from build123d import *

# Parameters (mm, degrees)
BOSS_EXTRUDE1_DEPTH = 8.89
CHAMFER1_SIZE       = 7.46
CHAMFER1_SIZE2      = 42.307762374


with BuildPart() as part:
    # Sketch2 → Boss-Extrude1 (new body)
    with BuildSketch(Plane(origin=(0, 0, 0), x_dir=(1, 0, 0), z_dir=(0, 1, 0))):
        Polygon((133.286430852, -770.74001749), (147.934191067, -816.056525657), (356.664774137, -778.521640105), (352.263248298, -717.230631168), align=None)
    extrude(amount=-BOSS_EXTRUDE1_DEPTH)

    # Chamfer1
    chamfer1_edges = [part.edges().sort_by_distance(p)[0] for p in [
        (252.299482602, 0, 797.289082881),
    ]]
    chamfer1_side = [part.faces().sort_by_distance(p)[0] for p in [
        (252.299482602, -4.445, 797.289082881),
    ]]
    chamfer(chamfer1_edges, length=CHAMFER1_SIZE, length2=CHAMFER1_SIZE2, reference=chamfer1_side[0])


solid = part.part
The model under review builds one solid part; all positions refer to its coordinate system, in mm. Round coordinates to 2 decimals unless told otherwise and drop trailing zeros. Loops run counter-clockwise (first coordinate to the right, second up) from the corner with the lowest first, then second, coordinate; pieces in that order, holes last. Notation, with made-up numbers: (-27.75, 21) -> (-16.75, 21) arc R12 cw to (-16.75, 25) -> close; hole circle Ø2 at (63.25, 38.25). An arc over 180 degrees is marked (long way). Write item = value, one per line. Start each with the question number.
Item 1: To check wall thickness, follow L1, parallel to Y at x = 193, z = 766; L2, parallel to Y at x = 281.5, z = 792; L3, parallel to Z at x = 171.5, y = -8.25. State the ranges of each line that lie inside material, in increasing order.
Item 2: Take a section at C-C on y = -6. Give the boundary of the cut face in (x, z).
Item 3: Insertion check: pin 1 (12 mm diameter, centred on x = 319.5, z = 797, fed in from +Y). The pin has a flat end and moves straight along its axis. Give the tip position at first contact, or say it passes through.
Item 4: Take a section at B-B on z = 758. Give the boundary of the cut face in (x, y).
Item 5: Take a section at A-A on x = 202.5. Give the boundary of the cut face in (y, z), plus the area to 3 significant figures.
Item 6: Take a section at D-D on z = 801. Give the boundary of the cut face in (x, y), plus the area to 3 significant figures.
Result:
q1.L1 = -8.89 to -0.18
q1.L2 = -8.89 to -7.45
q1.L3 = 761.4 to 811.82
q2.outline = (133.29, 770.74) -> (352.26, 717.23) -> (356.07, 770.22) -> (145.36, 808.11) -> close
q3.pin_1 = through
q4.outline = (185.42, -8.89) -> (355.19, -8.89) -> (355.19, -3.85) -> (231.74, 0) -> (185.42, 0) -> close
q5.outline = (-8.89, 753.83) -> (0, 753.83) -> (0, 763.26) -> (-7.46, 806.24) -> (-8.89, 806.24) -> close
q5.area = 306 mm²
q6.outline = (143.07, -8.89) -> (231.66, -8.89) -> (231.66, -7.46) -> (143.07, -4.7) -> close
q6.area = 249 mm²
